Part model, mm, in its own coordinate system. A direction names the side the tool comes from. Round coordinates to 2 decimals unless told otherwise and drop trailing zeros. Order: outer loops, then holes, each group sorted by start corner. A loop starts at its lowest first (then second) coordinate and runs counter-clockwise, first axis right, second up. Notation, with made-up numbers: (31, 25) -> (59, 25) arc R22 ccw to (59, 45) -> close; hole circle Ø5 at (27, 30). An arc over 180 degrees is marked (long way). Use CSV: the item, a comma, the result in double quotes.
```python
from build123d import *

# Parameters (mm, degrees)
F0_W     = 21
F0_H     = 21.7
F3_D     = 2.5
F3_DEPTH = 6
F3_TIP   = 0.7510757738
F4_R     = 2.5
F5_DEPTH = 11
F6_R     = 2.5
F7_DEPTH = 0.7


with BuildPart() as f1:
    # F0 (on Front) → F1 (revolve)
    with BuildSketch(Plane.XZ):
        with Locations((10.5, 10.85)):
            Rectangle(F0_W, F0_H)
    revolve(axis=Axis((0, 0, 10.85), (0, 0, 1)))

    # F3
    with Locations(Plane(origin=(0, 0, 0), x_dir=(1, 0, 0), z_dir=(0, 0, -1))):
        with Locations((0, 12.5), (0, 8), (-9.5, 0), (9.5, 0), (0, -8), (0, -12.5)):
            Hole(F3_D / 2, depth=F3_DEPTH)
            with Locations((0, 0, -(F3_DEPTH + F3_TIP / 2))):  # 118° drill point
                Cone(0, F3_D / 2, F3_TIP, mode=Mode.SUBTRACT)

    # F4 (on face) → F5 (join)
    with BuildSketch(Plane.XY.offset(21.7)):
        Circle(F4_R)
    extrude(amount=F5_DEPTH)

    # F6 (on face) → F7 (join)
    with BuildSketch(Plane(origin=(0, 0, 0), x_dir=(1, 0, 0), z_dir=(0, 0, -1))):
        Circle(F6_R)
    extrude(amount=F7_DEPTH)


solid = f1.part
```
(1) Drop flat-ended pins along their axis: P1, Ø1.5, axis at x = -5.5, z = 4.5, coming from the +Y side; P2, Ø2, axis at x = 0, y = 12.5, coming from the +Z side; P3, Ø1.5, axis at y = -15.5, z = 5, coming from the -X side. Give the stop position or say it passes through.
Reply:
P1,"y = 20.46"
P2,"z = 21.7"
P3,"x = -14.95"
(2) Which spindle directions (+Z, -Z, +X, -X, +Y, -Y) get a long thin tool onto all of the face, cutting with end or side? Do faces 4 (the face through (-0.54, -2.44, 27.12)), 5 (the face through (10.75, -0.05, 3.04)), 6 (the face through (20.03, 6.31, 11)). Say none if no direction does.
Reply:
face 4,"+Z"
face 5,"-Z"
face 6,"+Z, -Z"
(3) Cut at B-B, the plane y = -5. Give the cut face in (x, z).
Reply:
outline,"(-20.4, 0) -> (20.4, 0) -> (20.4, 21.7) -> (-20.4, 21.7) -> close"
(4) Cut at C-C, the plane x = -16. Give the cut face in (y, z).
Reply:
outline,"(-13.6, 0) -> (13.6, 0) -> (13.6, 21.7) -> (-13.6, 21.7) -> close"
(5) Cut at A-A, the plane z = 21. Give the cut face in (x, y).
Reply:
outline,"circle Ø42 at (0, 0)"
(6) Pull direction X, two halves, no side cores. Call faces 1 (the face through (0.2, 12.58, 6.62)), 2 (the face through (-0.54, 2.44, -0.35)), 3 (the face through (0, 0, -0.7)): released by +X, released by -X, zero draft, split by the parting line, or undercut.
Reply:
face 1,"undercut"
face 2,"split by the parting line"
face 3,"zero draft"
(7) Probe probe 1 along Y at (x, z) = (0, 4.7); probe 2 along Z at (x, y) = (9, 8.5); probe 3 along Y at (x, z) = (9, 4). List the from-to ranges inside material, lowest first. Write a range as [from, to].
Reply:
probe 1,"[-21, -13.75], [-11.25, -9.25], [-6.75, 6.75], [9.25, 11.25], [13.75, 21]"
probe 2,"[0, 21.7]"
probe 3,"[-18.97, -1.15], [1.15, 18.97]"
